Read the model definition and answer for the solid it produces. Units are mm, in the model's axes. A direction names the side the tool comes from. Round coordinates to 2 decimals unless told otherwise and drop trailing zeros. Loops run counter-clockwise (first coordinate to the right, second up) from the corner with the lowest first, then second, coordinate; pieces in that order, holes last. Notation, with made-up numbers: M -21,-21.5 L 1,-21.5 A27 cw 1,17.5 Z; hole C -26.75,-38.5 d2. An arc over 180 degrees is marked long. Write each question's results on one line, items separated by ' | '.
from build123d import *

# Parameters (mm, degrees)
SKETCH_1_W          = 120
SKETCH_1_H          = 120
EXTRUDE_1_DEPTH     = 67
SHELL_1_T           = -5
SKETCH_3_R          = 30
EXTRUDE_2_DEPTH     = 5
SKETCH_2_R          = 1.65
SKETCH_2_R_2        = 18.5
CUT_EXTRUDE_1_DEPTH = 181.676506497
EXTRUDE_START       = -3
SKETCH_4_R          = 18.5
SKETCH_4_R_2        = 13
EXTRUDE_3_DEPTH     = 3
FILLET_2_R          = 5
SKETCH_6_W          = 110
SKETCH_6_H          = 10
CUT_EXTRUDE_2_DEPTH = 5
SKETCH_8_W          = 110
SKETCH_8_H          = 5
EXTRUDE_4_DEPTH     = 57
SKETCH_9_R          = 4
EXTRUDE_5_DEPTH     = 57
SKETCH_10_R         = 1.9
CUT_EXTRUDE_3_DEPTH = 3.5
CUT_EXTRUDE_4_DEPTH = 185.347497949
FILLET_3_R          = 3
CHAMFER_1_SIZE      = 4
CHAMFER_2_SIZE      = 0.5


with BuildPart() as part:
    # 草图1 → 凸台-拉伸1 (new body)
    with BuildSketch(Plane(origin=(0, 0, 0), x_dir=(1, 0, 0), z_dir=(0, 1, 0))):
        with Locations((60, 60)):
            Rectangle(SKETCH_1_W, SKETCH_1_H)
    extrude(amount=EXTRUDE_1_DEPTH)

    # 抽壳1
    shell_1_openings = [part.faces().sort_by_distance(p)[0] for p in [
        (60, 0, -60),
    ]]
    offset(amount=SHELL_1_T, openings=shell_1_openings, kind=Kind.INTERSECTION)

    # 草图3 → 凸台-拉伸2 (add)
    with BuildSketch(Plane(origin=(0, 67, 0), x_dir=(1, 0, 0), z_dir=(0, 1, 0))):
        with Locations(Location((60, 60, 0), (0, 0, 270))):
            Circle(SKETCH_3_R)
    extrude(amount=EXTRUDE_2_DEPTH)

    # 草图2 → 切除-拉伸1 (cut, through all)
    with BuildSketch(Plane.XZ.offset(-62)):
        with Locations(Location((44.5, -44.5, 0), (0, 0, 270))):
            Circle(SKETCH_2_R)
        with Locations(Location((44.5, -75.5, 0), (0, 0, 270))):
            Circle(SKETCH_2_R)
        with Locations(Location((75.5, -44.5, 0), (0, 0, 270))):
            Circle(SKETCH_2_R)
        with Locations(Location((75.5, -75.5, 0), (0, 0, 270))):
            Circle(SKETCH_2_R)
        with Locations(Location((60, -60, 0), (0, 0, 270))):
            Circle(SKETCH_2_R_2)
    extrude(amount=-CUT_EXTRUDE_1_DEPTH, mode=Mode.SUBTRACT)

    # 草图4 → 凸台-拉伸3 (add)
    with BuildSketch(Plane(origin=(0, 72, 0), x_dir=(1, 0, 0), z_dir=(0, 1, 0)).offset(EXTRUDE_START)):
        with Locations(Location((60, 60, 0), (0, 0, 90))):
            Circle(SKETCH_4_R)
        with Locations(Location((60, 60, 0), (0, 0, 270))):
            Circle(SKETCH_4_R_2, mode=Mode.SUBTRACT)
    extrude(amount=EXTRUDE_3_DEPTH)

    # 圆角2
    fillet_2_edges = [part.edges().sort_by_distance(p)[0] for p in [
        (60, 67, -90),
    ]]
    fillet(fillet_2_edges, radius=FILLET_2_R - 0.0001)  # a hair under: the kernel refuses the full size

    # 草图6 → 切除-拉伸2 (cut)
    with BuildSketch(Plane(origin=(0, 67, 0), x_dir=(1, 0, 0), z_dir=(0, 1, 0))):
        with Locations((60, 10)):
            Rectangle(SKETCH_6_W, SKETCH_6_H)
        with Locations((60, 110)):
            Rectangle(SKETCH_6_W, SKETCH_6_H)
    extrude(amount=-CUT_EXTRUDE_2_DEPTH, mode=Mode.SUBTRACT)

    # 草图8 → 凸台-拉伸4 (add)
    with BuildSketch(Plane.XZ.offset(-62)):
        with Locations((60, -17.5)):
            Rectangle(SKETCH_8_W, SKETCH_8_H)
        with Locations((60, -102.5)):
            Rectangle(SKETCH_8_W, SKETCH_8_H)
    extrude(amount=EXTRUDE_4_DEPTH)

    # 草图9 → 凸台-拉伸5 (add)
    with BuildSketch(Plane.XZ.offset(-62)):
        with Locations((20, -20)):
            Circle(SKETCH_9_R)
        with Locations((20, -100)):
            Circle(SKETCH_9_R)
        with Locations((100, -100)):
            Circle(SKETCH_9_R)
        with Locations((100, -20)):
            Circle(SKETCH_9_R)
    extrude(amount=EXTRUDE_5_DEPTH)

    # 草图10 → 切除-拉伸3 (cut)
    with BuildSketch(Plane.XZ.offset(-5)):
        with Locations(Location((20, -100, 0), (0, 0, 270))):
            Circle(SKETCH_10_R)
        with Locations(Location((100, -100, 0), (0, 0, 270))):
            Circle(SKETCH_10_R)
        with Locations(Location((100, -20, 0), (0, 0, 270))):
            Circle(SKETCH_10_R)
        with Locations(Location((20, -20, 0), (0, 0, 270))):
            Circle(SKETCH_10_R)
    extrude(amount=-CUT_EXTRUDE_3_DEPTH, mode=Mode.SUBTRACT)

    # 草图12 → 切除-拉伸4 (cut, through all)
    with BuildSketch(Plane(origin=(120, 0, 0), x_dir=(0, 0, -1), z_dir=(1, 0, 0))):
        Polygon((31.5, 58.464466094), (56.464466094, 33.5), (31.5, 8.535533906), align=None)
        Polygon((35.035533906, 62), (84.964466094, 62), (60, 37.035533906), align=None)
        Polygon((88.5, 58.464466094), (88.5, 8.535533906), (63.535533906, 33.5), align=None)
        Polygon((84.964466094, 5), (35.035533906, 5), (60, 29.964466094), align=None)
    extrude(amount=-CUT_EXTRUDE_4_DEPTH, mode=Mode.SUBTRACT)

    # 圆角3
    fillet_3_edges = [part.edges().sort_by_distance(p)[0] for p in [
        (2.5, 33.5, -63.535533906),
        (2.5, 58.464466094, -88.5),
        (2.5, 8.535533906, -88.5),
        (117.5, 33.5, -63.535533906),
        (117.5, 58.464466094, -88.5),
        (117.5, 8.535533906, -88.5),
        (2.5, 37.035533906, -60),
        (2.5, 62, -84.964466094),
        (2.5, 62, -35.035533906),
        (117.5, 62, -35.035533906),
        (117.5, 37.035533906, -60),
        (117.5, 62, -84.964466094),
        (2.5, 29.964466094, -60),
        (2.5, 5, -84.964466094),
        (2.5, 5, -35.035533906),
        (117.5, 29.964466094, -60),
        (117.5, 5, -84.964466094),
        (117.5, 5, -35.035533906),
        (2.5, 8.535533906, -31.5),
        (2.5, 58.464466094, -31.5),
        (2.5, 33.5, -56.464466094),
        (117.5, 8.535533906, -31.5),
        (117.5, 58.464466094, -31.5),
        (117.5, 33.5, -56.464466094),
    ]]
    fillet(fillet_3_edges, radius=FILLET_3_R)

    # 倒角1
    chamfer_1_edges = [part.edges().sort_by_distance(p)[0] for p in [
        (120, 67, -60),
        (60, 67, -120),
        (0, 67, -60),
        (60, 67, -15),
        (60, 67, -105),
        (0, 33.5, -120),
        (120, 33.5, -120),
        (120, 33.5, 0),
        (0, 33.5, 0),
        (60, 67, 0),
    ]]
    chamfer(chamfer_1_edges, length=CHAMFER_1_SIZE)

    # 倒角2
    chamfer_2_edges = [part.edges().sort_by_distance(p)[0] for p in [
        (20, 5, -18.1),
        (100, 5, -18.1),
        (100, 5, -98.1),
        (20, 5, -98.1),
    ]]
    chamfer(chamfer_2_edges, length=CHAMFER_2_SIZE)


solid = part.part
Item 1: Straight lines are drawn through the part: line 1 (Z direction, x = 106, y = 26.5); line 2 (X direction, y = 69.5, z = -44.5); line 3 (Z direction, x = 75.5, y = 64.5). For each, find the intervals that lie inside material, in ascending order.
Outcome:
line 1: z = -120 to -115, -105 to -100, -20 to -15, -5 to 0 | line 2: x = 33.54 to 42.85, 46.15 to 73.85, 77.15 to 86.46 | line 3: z = -118.5 to -115, -103.5 to -77.15, -73.85 to -70.1, -49.9 to -46.15, -42.85 to -16.5, -5 to -1.5
Item 2: The part is cut by section A-A (x = 12). Determine the outline of the cut face in (y, z), plus the area to 3 significant figures.
Outcome:
outline: M 0,-120 L 63,-120 L 67,-116 L 67,-115 L 0,-115 Z; M 0,-5 L 67,-5 L 67,-4 L 63,0 L 0,0 Z; M 5,-105 L 63,-105 L 67,-101 L 67,-19 L 63,-15 L 5,-15 L 5,-20 L 62,-20 L 62,-100 L 5,-100 Z | area: 1,660 mm2
Item 3: Flat-ended cylindrical pins translate along their axes: pin 1 (4 mm diameter, centred on x = 75.5, z = -75.5, fed in from -Y); pin 2 (4 mm diameter, centred on x = 15.5, z = -66, fed in from +Y); pin 3 (4.5 mm diameter, centred on x = 52.5, z = -99.5, fed in from -Y). Find the tip coordinate at first contact, or state that the pin passes through.
Outcome:
pin 1: stops at y = 62 | pin 2: stops at y = 67 | pin 3: stops at y = 5
Item 4: For faces 1 (the face through (59, 34, -115)), 2 (the face through (118, 65, -59)), 3 (the face through (59, 34, -100)), 4 (the face through (0, 31, -59)), 5 (the face through (3, 33, -31.5)), determine the directions among +Z, -Z, +X, -X, +Y, -Y from which every point of the face is accessible in a straight line to the end or side of a thin tool.
Outcome:
face 1: +Y, -Y | face 2: +Z, -Z, +X, +Y | face 3: -Y | face 4: +Z, -Z, -X, +Y, -Y | face 5: +X, -X
Item 5: The mould has two halves that part along Z. Classify faces 6 (the face through (2.465, 13.026, -33.306)), 7 (the face through (2, 65, -59)), 8 (the face through (118, 31, -118)): pulls with the +Z half, pulls with the -Z half, needs draft (parallel to the pull), parting line crosses it, or undercut.
Outcome:
face 6: undercut | face 7: needs draft | face 8: pulls with the -Z half
Item 6: The part is cut by section B-B (x = 60). State how many separate pieces and enclosed holes the cut face has, plus the area to 3 significant figures.
Outcome:
separate pieces: 4 | enclosed holes: 0 | area: 1,630 mm2
